Check sheet for the modelled part. Datum: model origin and axes. Units: mm. Face numbers are marked on the shaded views. Give positions to 0.01 mm unless a question says otherwise; leave off trailing zeros. Loops run counter-clockwise (first coordinate to the right, second up) from the corner with the lowest first, then second, coordinate; pieces in that order, holes last. Notation, with made-up numbers: (28, 25) -> (82, 25) arc R19 ccw to (82, 47) -> close; hole circle Ø3 at (-16.75, 27.5). An arc over 180 degrees is marked (long way). Answer as CSV lines item,"result". Start each with the question number.
(1) Material ranges on line 1 (X direction, y = 273, z = -19) (3 decimals); line 2 (Z direction, x = 50.5, y = 199) (3 decimals); line 3 (X direction, y = -293.5, z = -33.5) (3 decimals), recorded low to high. Write a range as from..to.
(2) Gauge pin test, flat ends, axial feed: pin 1 Ø6 at (x, y) = (15, -272) entering from +Z; pin 2 Ø6 at (x, y) = (81.5, 318) entering from +Z (3 decimals). Record the tip position at first contact, or that the pin passes through.
(3) Section check B-B on y = -163. Enter the section's corners in (x, z) (3 decimals), plus the area to 3 significant figures.
(4) Section check A-A on z = -19. Enter the section's corners in (x, y) (3 decimals).
(5) Release check for a two-part mould opening along X. For the marked faces 1, 2 and 3 record: pulls with the +X half, pulls with the -X half, needs draft (parallel to the pull), parting line crosses it, or undercut.
(6) Section check C-C on x = 54.5. Enter the section's corners in (y, z) (3 decimals), plus the area to 3 significant figures.
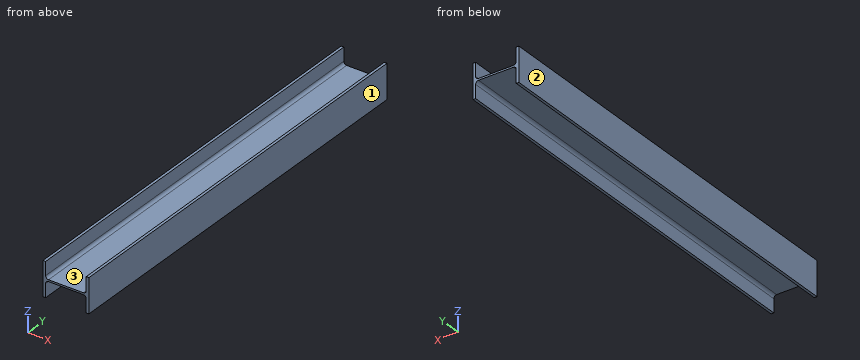
from build123d import *

# Parameters (mm, degrees)
AL_I_BEAM_AL_I_BEAM_4X2_31_1_DEPTH = 914.4


with BuildPart() as part:
    # Sketch11 → Al i beam AL I BEAM 4X2.31(1) (new body)
    with BuildSketch(Plane(origin=(53.975, -457.2, -38.1), x_dir=(0, 0, -1), z_dir=(0, 1, 0))):
        with BuildLine():
            Line((-38.1, -50.8), (-38.1, -44.958))
            Line((-38.1, -44.958), (-8.255, -44.958))
            ThreePointArc((-8.255, -44.958), (-3.764871939, -43.098128061), (-1.905, -38.608))
            Line((-1.905, -38.608), (-1.905, 38.608))
            ThreePointArc((-1.905, 38.608), (-3.764871939, 43.098128061), (-8.255, 44.958))
            Line((-8.255, 44.958), (-38.1, 44.958))
            Line((-38.1, 44.958), (-38.1, 50.8))
            Line((-38.1, 50.8), (38.1, 50.8))
            Line((38.1, 50.8), (38.1, 44.958))
            Line((38.1, 44.958), (8.255, 44.958))
            ThreePointArc((8.255, 44.958), (3.764871939, 43.098128061), (1.905, 38.608))
            Line((1.905, 38.608), (1.905, -38.608))
            ThreePointArc((1.905, -38.608), (3.764871939, -43.098128061), (8.255, -44.958))
            Line((8.255, -44.958), (38.1, -44.958))
            Line((38.1, -44.958), (38.1, -50.8))
            Line((38.1, -50.8), (-38.1, -50.8))
        make_face()
    extrude(amount=AL_I_BEAM_AL_I_BEAM_4X2_31_1_DEPTH)


solid = part.part
Working result:
1,line 1,"x = 3.175..9.017, 98.933..104.775"
1,line 2,"z = -40.005..-36.195"
1,line 3,"x = 3.175..10.174, 97.776..104.775"
2,pin 1,"stops at z = -35.23"
2,pin 2,"stops at z = -36.195"
3,outline,"(3.175, -76.2) -> (9.017, -76.2) -> (9.017, -46.355) arc R6.35 cw to (15.367, -40.005) -> (92.583, -40.005) arc R6.35 cw to (98.933, -46.355) -> (98.933, -76.2) -> (104.775, -76.2) -> (104.775, 0) -> (98.933, 0) -> (98.933, -29.845) arc R6.35 cw to (92.583, -36.195) -> (15.367, -36.195) arc R6.35 cw to (9.017, -29.845) -> (9.017, 0) -> (3.175, 0) -> close"
3,area,"1,270 mm^2"
4,outline,"(3.175, -457.2) -> (9.017, -457.2) -> (9.017, 457.2) -> (3.175, 457.2) -> close; (98.933, -457.2) -> (104.775, -457.2) -> (104.775, 457.2) -> (98.933, 457.2) -> close"
5,face 1,"pulls with the +X half"
5,face 2,"pulls with the -X half"
5,face 3,"undercut"
6,outline,"(-457.2, -40.005) -> (457.2, -40.005) -> (457.2, -36.195) -> (-457.2, -36.195) -> close"
6,area,"3,480 mm^2"
